```python
from build123d import *

# Parameters (mm, degrees)
F1_DEPTH = 70
F2_SIZE2 = 0.36396
F2_SIZE  = 0.99999
F4_D     = 0.2
F4_DEPTH = 0.9
F4_TIP   = 0.0600860619


# Not quite as in the source:
# - a fillet or chamfer is up to 0.001 mm smaller than in the source, because OpenCascade refuses the exact size


with BuildPart() as f1:
    # F0 (on Right) → F1 (new body)
    with BuildSketch(Plane.YZ):
        Polygon((-39.5598503354, -13.8284793004), (-40.5598503354, -13.8284793004), (-40.5598503354, -18.5284793004), (-41.0598503354, -18.5284793004), (-41.0598503354, -19.5284793004), (-39.5598503354, -19.5284793004), align=None)
    extrude(amount=-F1_DEPTH)

    # F2 (size 1 and 0.3639702343 in the source; OpenCascade refuses exactly that, so slightly less here)
    f2_edges = [f1.edges().sort_by_distance(p)[0] for p in [
        (-35, -39.55985, -13.828479),
    ]]
    f2_side = f1.faces().sort_by_distance((-35, -40.05985, -13.828479))[0]
    chamfer(f2_edges, length=F2_SIZE, length2=F2_SIZE2, reference=f2_side)

    # F4
    with Locations(Plane.XZ.offset(40.5598503354)):
        with Locations((-62.5, -14.7784793004), (-60.8, -14.7784793004), (-59.1, -14.7784793004), (-10.9, -14.7784793004), (-9.2, -14.7784793004), (-7.5, -14.7784793004)):
            Hole(F4_D / 2, depth=F4_DEPTH)
            with Locations((0, 0, -(F4_DEPTH + F4_TIP / 2))):  # 118° drill point
                Cone(0, F4_D / 2, F4_TIP, mode=Mode.SUBTRACT)


solid = f1.part
```
Here's how the part is built. I have some questions about the finished solid (model axes, mm). A direction names the side the tool comes from. Give positions to 0.01 mm unless a question says otherwise; leave off trailing zeros. Order: outer loops, then holes, each group sorted by start corner. A loop starts at its lowest first (then second) coordinate and runs counter-clockwise, first axis right, second up. Notation, with made-up numbers: (-11, 83.5) -> (20, 83.5) arc R8 ccw to (20, 96.5) -> close; hole circle Ø4 at (65, -7). An arc over 180 degrees is marked (long way). Use CSV: the item, a comma, the result in double quotes. Start each with the question number.
Item 1: Suppose I cut it at B-B (y = -40.1). List the corners of the cut face in (x, z) for me.
Item 2: On a 3-axis mill with a long thin cutter (end or side, diameter ignored), from which of +Z, -Z, +X, -X, +Y, -Y can I reach the whole of each face in a straight line? I mean faces 1 (the flat face through (-35, -40, -19.528)), 2 (the flat face through (-35, -40.56, -16)). Say none if no direction works.
Item 3: If I drill on probe 1 along Y at (x, z) = (-47.5, -16.65); probe 2 along Z at (x, y) = (-62.5, -40.3); probe 3 along Z at (x, y) = (-10.9, -40.15), over which ranges is the centre line in solid material (lowest first)? Write a range as [from, to].
Item 4: Suppose I cut it at C-C (z = -17.6). List the corners of the cut face in (x, y) for me.
Answer block:
1,outline,"(-70, -19.53) -> (0, -19.53) -> (0, -14) -> (-70, -14) -> close; hole circle Ø0.2 at (-62.5, -14.78); hole circle Ø0.2 at (-60.8, -14.78); hole circle Ø0.2 at (-59.1, -14.78); hole circle Ø0.2 at (-10.9, -14.78); hole circle Ø0.2 at (-9.2, -14.78); hole circle Ø0.2 at (-7.5, -14.78)"
2,face 1,"-Z, +X, -X, +Y, -Y"
2,face 2,"+Z, +X, -X, -Y"
3,probe 1,"y = [-40.56, -39.56]"
3,probe 2,"z = [-19.53, -14.88], [-14.68, -13.92]"
3,probe 3,"z = [-19.53, -14.88], [-14.68, -13.98]"
4,outline,"(-70, -40.56) -> (0, -40.56) -> (0, -39.56) -> (-70, -39.56) -> close"
